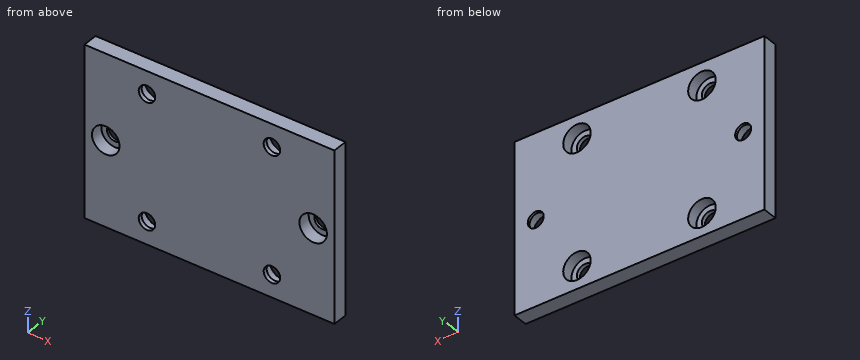
Autodesk Inventor part; units mm, degrees
ref_plane "YZ Plane" through (0, 0, 0) normal (1, 0, 0) x (0, 1, 0)
ref_plane "XZ Plane" through (0, 0, 0) normal (0, 1, 0) x (-1, 0, 0)
ref_plane "XY Plane" through (0, 0, 0) normal (0, 0, 1) x (1, 0, 0)
sketch "Sketch1" plane through (0, 0, 0) normal (0, 1, 0) x (-1, 0, 0)
  line L0 (-50, 34) -> (50, 34)
  line L1 (50, 34) -> (50, -34)
  line L2 (50, -34) -> (-50, -34)
  line L3 (-50, -34) -> (-50, 34)
  line L4 (-50, 34) -> (50, -34) construction
  line L5 (50, 34) -> (-50, -34) construction
  point P0 (0, 0)
  dimension "d0" = 68
  dimension "d1" = 100
extrude "Extrusion1" add sketch "Sketch1" along normal blind 6
sketch "Sketch2" plane through (0, 0, 0) normal (0, 1, 0) x (1, 0, 0)
  line L0 (0, 47.6) -> (0, -47.6)
  point P0 (0, 0)
  point P1 (-41.5, 0)
  point P2 (41.5, 0)
  dimension "d4" = 83
sketch "Sketch3" plane through (0, 6, 0) normal (0, 1, 0) x (1, 0, 0)
  line L0 (25, 25) -> (-25, 25) construction
  line L1 (-25, 25) -> (-25, -25) construction
  line L2 (-25, -25) -> (25, -25) construction
  line L3 (25, -25) -> (25, 25) construction
  line L4 (25, 25) -> (-25, -25) construction
  line L5 (-25, 25) -> (25, -25) construction
  point P0 (0, 0)
  dimension "d12" = 50
  dimension "d13" = 50
hole "Hole2" at (-25, 6, 25) at (-25, 6, -25) at (25, 6, -25) at (25, 6, 25) direction (0, -1, 0) diameter 6.6 end through all counterbore diameter 11 counterbore depth 4.4
hole "Hole3" at (-41.5, 0, 0) at (41.5, 0, 0) direction (0, 1, 0) diameter 6.4 end through all counterbore diameter 11 counterbore depth 5
properties part number "KN-00-01-02" material "X5CrNi18-10"
Can you work these out from the model? Positions are in its coordinate system, mm. Give positions to 0.01 mm unless a question says otherwise; leave off trailing zeros. Order: outer loops, then holes, each group sorted by start corner. A loop starts at its lowest first (then second) coordinate and runs counter-clockwise, first axis right, second up. Notation, with made-up numbers: M 50.5,-23 L 73.5,-23 A15 ccw 73.5,-4 Z; hole C -33,-32.5 d3. An arc over 180 degrees is marked long. One line per question, with ' | ' between items.
Item 1: Suppose I cut it at C-C, the plane y = 2.5. Write out the boundary of the cut face in (x, z).
Answer block:
outline: M -50,-34 L 50,-34 L 50,34 L -50,34 Z; hole C -41.5,0 d11; hole C -25,-25 d11; hole C -25,25 d11; hole C 25,-25 d11; hole C 25,25 d11; hole C 41.5,0 d11
Item 2: I'm going to push flat-ended pins straight in: pin 1 Ø7.5 at (x, z) = (-25, 25) entering from +Y; pin 2 Ø17.5 at (x, z) = (-25, -25) entering from -Y; pin 3 Ø5.5 at (x, z) = (-25, -25) entering from -Y; pin 4 Ø8.5 at (x, z) = (41.5, 0) entering from -Y. Where does each tip first touch, or does it pass through?
Answer block:
pin 1: stops at y = 1.6 | pin 2: stops at y = 0 | pin 3: passes through | pin 4: stops at y = 5
Item 3: Suppose I cut it at A-A, the plane z = -25. Write out the boundary of the cut face in (x, y).
Answer block:
outline: M -50,0 L -28.3,0 L -28.3,1.6 L -30.5,1.6 L -30.5,6 L -50,6 Z; M -21.7,0 L 21.7,0 L 21.7,1.6 L 19.5,1.6 L 19.5,6 L -19.5,6 L -19.5,1.6 L -21.7,1.6 Z; M 28.3,0 L 50,0 L 50,6 L 30.5,6 L 30.5,1.6 L 28.3,1.6 Z
Item 4: Suppose I cut it at D-D, the plane x = 25. Write out the boundary of the cut face in (y, z).
Answer block:
outline: M 0,-34 L 6,-34 L 6,-30.5 L 1.6,-30.5 L 1.6,-28.3 L 0,-28.3 Z; M 0,-21.7 L 1.6,-21.7 L 1.6,-19.5 L 6,-19.5 L 6,19.5 L 1.6,19.5 L 1.6,21.7 L 0,21.7 Z; M 0,28.3 L 1.6,28.3 L 1.6,30.5 L 6,30.5 L 6,34 L 0,34 Z
Item 5: Suppose I cut it at B-B, the plane x = 41.5. Write out the boundary of the cut face in (y, z), then the cut area to 3 significant figures.
Answer block:
outline: M 0,-34 L 6,-34 L 6,-3.2 L 5,-3.2 L 5,-5.5 L 0,-5.5 Z; M 0,5.5 L 5,5.5 L 5,3.2 L 6,3.2 L 6,34 L 0,34 Z | area: 347 mm2
Item 6: Please list where these lines run through material, in increasing order: L1, parallel to Z at x = -25, y = 2.9; L2, parallel to Z at x = 25, y = 0.7; L3, parallel to X at y = 2.3, z = 0.
Answer block:
L1: z = -34 to -30.5, -19.5 to 19.5, 30.5 to 34 | L2: z = -34 to -28.3, -21.7 to 21.7, 28.3 to 34 | L3: x = -50 to -47, -36 to 36, 47 to 50
